Can you work these out from the model? Positions are in its coordinate system, mm. A direction names the side the tool comes from. Coordinates: 2 decimals unless noted, no trailing zeros. Order: outer loops, then holes, each group sorted by start corner. A loop starts at its lowest first (then second) coordinate and runs counter-clockwise, first axis right, second up. Notation, with made-up numbers: (48, 88) -> (60, 88) arc R14 cw to (60, 103) -> close; hole circle Ø9 at (83.5, 5.5). An arc over 180 degrees is marked (long way). Answer in a Markdown table with one row per item.
```python
from build123d import *

# Parameters (mm, degrees)
THICKEN1_START           = -92.5
THICKEN1_OUTLINE_W       = 30
THICKEN1_OUTLINE_H       = 4.5
THICKEN1_DEPTH           = 185
THICKEN2_START           = -92.5
THICKEN2_OUTLINE_W       = 3
THICKEN2_OUTLINE_H       = 18
THICKEN2_DEPTH           = 185
THICKEN3_START           = -92.5
THICKEN3_OUTLINE_W       = 3
THICKEN3_OUTLINE_H       = 18
THICKEN3_DEPTH           = 185
BOSS_EXTRUDE1_DEPTH      = 185
SKETCH7_W                = 36
SKETCH7_H                = 8
CUT_EXTRUDE1_DEPTH       = 187.604528348
BOSS_EXTRUDE2_DEPTH      = 7.5
BOSS_EXTRUDE3_START      = 7.5
BOSS_EXTRUDE3_DEPTH      = 7.5
BOSS_EXTRUDE4_DEPTH      = 9.5
BOSS_EXTRUDE4_DEPTH_BACK = 9.5
SKETCH10_R               = 6
SKETCH10_R_2             = 2
BOSS_EXTRUDE5_DEPTH      = 3
BOSS_EXTRUDE5_DEPTH_BACK = 3
SKETCH11_R               = 6
SKETCH11_R_2             = 2


# Read off the part's stored shape, not the designer's step: Thicken1, Thicken2, Thicken3
with BuildPart() as part:
    # Thicken1 outline → Thicken1 (new body)
    with BuildSketch(Plane.XY.offset(THICKEN1_START)):
        with Locations((0, 0.75)):
            Rectangle(THICKEN1_OUTLINE_W, THICKEN1_OUTLINE_H)
    extrude(amount=THICKEN1_DEPTH)

    # Thicken2 outline → Thicken2 (add)
    with BuildSketch(Plane.XY.offset(THICKEN2_START)):
        with Locations((16.5, 7.5)):
            Rectangle(THICKEN2_OUTLINE_W, THICKEN2_OUTLINE_H)
    extrude(amount=THICKEN2_DEPTH)

    # Thicken3 outline → Thicken3 (add)
    with BuildSketch(Plane.XY.offset(THICKEN3_START)):
        with Locations((-16.5, 7.5)):
            Rectangle(THICKEN3_OUTLINE_W, THICKEN3_OUTLINE_H)
    extrude(amount=THICKEN3_DEPTH)

    # Sketch4 → Boss-Extrude1 (add)
    with BuildSketch(Plane.XY.offset(92.5)):
        with BuildLine():
            Line((-15, 16.5), (-15, 3))
            Line((-15, 3), (15, 3))
            Line((15, 3), (15, 16.5))
            ThreePointArc((15, 16.5), (0, 9.728756555), (-15, 16.5))
        make_face()
    extrude(amount=-BOSS_EXTRUDE1_DEPTH)

    # Sketch7 → Cut-Extrude1 (cut, through all)
    with BuildSketch(Plane(origin=(0, 0, -92.5), x_dir=(-1, 0, 0), z_dir=(0, 0, -1))):
        with Locations((0, 2.5)):
            Rectangle(SKETCH7_W, SKETCH7_H)
    extrude(amount=-CUT_EXTRUDE1_DEPTH, mode=Mode.SUBTRACT)

    # Sketch8 → Boss-Extrude2 (add)
    with BuildSketch(Plane(origin=(0, 0, -92.5), x_dir=(-1, 0, 0), z_dir=(0, 0, -1))):
        with BuildLine():
            Line((-18, 6.5), (18, 6.5))
            Line((18, 6.5), (18, 16.5))
            Line((18, 16.5), (15, 16.5))
            ThreePointArc((15, 16.5), (0, 9.728756555), (-15, 16.5))
            Line((-15, 16.5), (-18, 16.5))
            Line((-18, 16.5), (-18, 6.5))
        make_face()
    extrude(amount=BOSS_EXTRUDE2_DEPTH)

    # Sketch9 → Boss-Extrude3 (add)
    with BuildSketch(Plane.XY.offset(92.5).offset(BOSS_EXTRUDE3_START)):
        with BuildLine():
            Line((-18, 6.5), (18, 6.5))
            Line((18, 6.5), (18, 16.5))
            Line((18, 16.5), (15, 16.5))
            ThreePointArc((15, 16.5), (0, 9.728756555), (-15, 16.5))
            Line((-15, 16.5), (-18, 16.5))
            Line((-18, 16.5), (-18, 6.5))
        make_face()
    extrude(amount=-BOSS_EXTRUDE3_DEPTH)

    # Sketch10 → Boss-Extrude4 (add, two sides: drawn at the far end of the back side and taken through both)
    # profile 1 of 2: a face of its own
    with BuildSketch(Plane(origin=(0, 0, 0), x_dir=(0, 0, -1), z_dir=(1, 0, 0)).offset(-BOSS_EXTRUDE4_DEPTH_BACK)):
        Circle(SKETCH10_R)
        Circle(SKETCH10_R_2, mode=Mode.SUBTRACT)
    # profile 2 of 2: a face of its own
    with BuildSketch(Plane(origin=(0, 0, 0), x_dir=(0, 0, -1), z_dir=(1, 0, 0)).offset(-BOSS_EXTRUDE4_DEPTH_BACK)):
        with BuildLine():
            Line((10, 6.5), (-10, 6.5))
            Line((-10, 6.5), (-5.35678593, -2.702747584))
            ThreePointArc((-5.35678593, -2.702747584), (-1.389115622, 5.836981908), (6, 0))
            ThreePointArc((6, 0), (5.836981908, -1.389115622), (5.35678593, -2.702747584))
            Line((5.35678593, -2.702747584), (10, 6.5))
        make_face()
    extrude(amount=BOSS_EXTRUDE4_DEPTH + BOSS_EXTRUDE4_DEPTH_BACK)

    # Sketch11 → Boss-Extrude5 (add, two sides: drawn at the far end of the back side and taken through both)
    # profile 1 of 2: a face of its own
    with BuildSketch(Plane(origin=(0, 0, 0), x_dir=(0, 0, -1), z_dir=(1, 0, 0)).offset(-BOSS_EXTRUDE5_DEPTH_BACK)):
        with Locations((92.5, 0)):
            Circle(SKETCH11_R)
        with Locations(Location((92.5, 0, 0), (0, 0, 90))):
            Circle(SKETCH11_R_2, mode=Mode.SUBTRACT)
    # profile 2 of 2: a face of its own
    with BuildSketch(Plane(origin=(0, 0, 0), x_dir=(0, 0, -1), z_dir=(1, 0, 0)).offset(-BOSS_EXTRUDE5_DEPTH_BACK)):
        with BuildLine():
            ThreePointArc((86.5, 0), (92.5, 6), (98.5, 0))
            Line((98.5, 0), (98.5, 6.5))
            Line((98.5, 6.5), (86.5, 6.5))
            Line((86.5, 6.5), (86.5, 0))
        make_face()
    extrude(amount=BOSS_EXTRUDE5_DEPTH + BOSS_EXTRUDE5_DEPTH_BACK)


solid = part.part
```
(1) I need wall thicknesses on line 1 (Y direction, x = 1.25, z = 0); line 2 (X direction, y = 15.75, z = 3.5); line 3 (Y direction, x = 0, z = -92). Which ranges of each line are inside material? Lowest first, please. Write a range as [from, to].
Response values:
| item | result |
|---|---|
| line 1 | [-6, -2], [2, 9.77] |
| line 2 | [-18, -14.3], [14.3, 18] |
| line 3 | [-5.98, -1.94], [1.94, 9.73] |
(2) Suppose I cut it at D-D (x = 1). Please give me the cut outline in (y, z), and give its area (3 significant figures).
Response values:
| item | result |
|---|---|
| outline | (-2.7, -5.36) -> (6.5, -10) -> (6.5, -86.5) -> (0, -86.5) arc R6 ccw to (0, -98.5) -> (6.5, -98.5) -> (6.5, -100) -> (9.75, -100) -> (9.75, 100) -> (6.5, 100) -> (6.5, 10) -> (-2.7, 5.36) arc R6 ccw to start; hole circle Ø4 at (0, -92.5); hole circle Ø4 at (0, 0) |
| area | 927 mm2 |
(3) On a 3-axis mill with a long thin cutter (end or side, diameter ignored), from which of +Z, -Z, +X, -X, +Y, -Y can I reach the whole of each face in a straight line? I mean faces 1 (the flat face through (3, 2, -91)), 2 (the flat face through (0, 3, -86.5)), 3 (the flat face through (9.5, 3, 0)), 4 (the flat face through (0, 3, -98.5)). Say none if no direction works.
Response values:
| item | result |
|---|---|
| face 1 | -Z, +X, -Y |
| face 2 | +X, -X, -Y |
| face 3 | +Z, -Z, +X, -Y |
| face 4 | -Z, +X, -X, -Y |
(4) Suppose I cut it at A-A (z = -92.5). Please give me the cut outline in (x, y).
Response values:
| item | result |
|---|---|
| outline | (-18, 6.5) -> (-3, 6.5) -> (-3, 2) -> (3, 2) -> (3, 6.5) -> (18, 6.5) -> (18, 16.5) -> (15, 16.5) arc R20 cw to (-15, 16.5) -> (-18, 16.5) -> close; (-3, -6) -> (3, -6) -> (3, -2) -> (-3, -2) -> close |
(5) Suppose I cut it at B-B (y = 12.25). Please give me the cut outline in (x, z), and give its area (3 significant figures).
Response values:
| item | result |
|---|---|
| outline | (-18, -100) -> (-9.72, -100) -> (-9.72, 100) -> (-18, 100) -> close; (9.72, -100) -> (18, -100) -> (18, 100) -> (9.72, 100) -> close |
| area | 3,310 mm2 |
(6) Suppose I cut it at C-C (z = -43). Please give me the cut outline in (x, y).
Response values:
| item | result |
|---|---|
| outline | (-18, 6.5) -> (18, 6.5) -> (18, 16.5) -> (15, 16.5) arc R20 cw to (-15, 16.5) -> (-18, 16.5) -> close |
(7) Will these pins go through, and if not, where does the flat tip stop? pin 1 Ø1 at (x, z) = (7, 20.5) entering from +Y; pin 2 Ø10 at (y, z) = (0.5, 0.5) entering from +X; pin 3 Ø1 at (x, z) = (-3.5, 64.5) entering from -Y; pin 4 Ø1.5 at (y, z) = (2.5, 10) entering from +X.
Response values:
| item | result |
|---|---|
| pin 1 | y = 11.19 |
| pin 2 | x = 9.5 |
| pin 3 | y = 6.5 |
| pin 4 | through |
(8) We'd pull the mould along X, two halves only. Please class faces 5 (the cylindrical face through (0.24, 9.73, 1.4)), 6 (the flat face through (-9.5, 3, 0)), 7 (the flat face through (0, 9, -100)): +X half, -X half, draft (parallel to the pull), parting line (faces both ways), or undercut.
Response values:
| item | result |
|---|---|
| face 5 | undercut |
| face 6 | -X half |
| face 7 | draft |
